Design review of the part built by this model. Coordinates are the model's own, in mm. A direction names the side the tool comes from. Coordinates: 2 decimals unless noted, no trailing zeros. Write each loop counter-clockwise with the first axis right and the second up, starting at its lowest first coordinate (ties: lowest second). Pieces come first, ordered by that corner, then holes. Notation, with made-up numbers: M 88.5,15 L 139.5,15 A20 cw 139.5,27 Z; hole C 13.25,52.5 d6. An arc over 180 degrees is marked long. Write item = value, one per line.
```python
from build123d import *

# Parameters (mm, degrees)
SKETCH001_R   = 8
PAD_DEPTH     = 4.05
SKETCH002_R   = 9.892347
SKETCH002_R_2 = 8.778396
PAD001_DEPTH  = 4.825


with BuildPart() as part:
    # Sketch001 → Pad (new body, symmetric)
    with BuildSketch(Plane.XY):
        with BuildLine():
            ThreePointArc((-12.471576, -8.239007), (5.253972, -13.993471), (14.812215, 2.004932))
            ThreePointArc((14.049591, 4.890442), (13.918155, 3.312171), (14.812215, 2.004932))
            ThreePointArc((14.049591, 4.890442), (6.504678, 10.917918), (-3.152003, 10.849328))
            ThreePointArc((-10.894672, 13.052776), (-7.942462, 8.721353), (-3.152003, 10.849328))
            Line((-10.894672, 13.052776), (-12.022041, 13.052776))
            Line((-12.022041, 13.052776), (-17.151012, 7.540552))
            Line((-17.151012, 7.540552), (-57.172882, 8.741419))
            Line((-83.948982, -1.605249), (-57.172882, 8.741419))
            Line((-82.650063, -5.462648), (-83.948982, -1.605249))
            Line((-57.419521, 2.370234), (-82.650063, -5.462648))
            Line((-20.377901, -5.481424), (-57.419521, 2.370234))
            Line((-18.078703, -9.566922), (-20.377901, -5.481424))
            Line((-12.471576, -8.239007), (-18.078703, -9.566922))
        make_face()
        Circle(SKETCH001_R, mode=Mode.SUBTRACT)
    extrude(amount=PAD_DEPTH, both=True)

    # Sketch002 → Pad001 (join, symmetric)
    with BuildSketch(Plane.XY):
        Circle(SKETCH002_R)
        Circle(SKETCH002_R_2, mode=Mode.SUBTRACT)
    extrude(amount=PAD001_DEPTH, both=True)


solid = part.part
```
Q1. For P1, Ø3, axis at y = -5, z = -1, coming from the +X side; P2, Ø5.5, axis at x = 2, y = -3.5, coming from the +Z side; P3, Ø5, axis at x = -5.5, z = 4, coming from the -Y side; P4, Ø2, axis at x = -57.5, z = 3.5, coming from the -Y side, all flat-tipped, find the tip position at first contact; note any pin that passes through.
Check result:
P1 = 14.53
P2 = through
P3 = -14.64
P4 = 2.03
Q2. Consider section D-D, the plane x = 0. State the section outline as (y, z) points (3 decimals), and give its area (3 significant figures).
Check result:
outline = M -14.947,-4.05 L -9.892,-4.05 L -9.892,-4.825 L -8.778,-4.825 L -8.778,-4.05 L -8,-4.05 L -8,4.05 L -8.778,4.05 L -8.778,4.825 L -9.892,4.825 L -9.892,4.05 L -14.947,4.05 Z; M 8,-4.05 L 8.778,-4.05 L 8.778,-4.825 L 9.892,-4.825 L 9.892,-4.05 L 11.605,-4.05 L 11.605,4.05 L 9.892,4.05 L 9.892,4.825 L 8.778,4.825 L 8.778,4.05 L 8,4.05 Z
area = 88.9 mm²
Q3. Consider section B-B, the plane y = 0. State the section outline as (x, z) points (3 decimals).
Check result:
outline = M -79.795,-4.05 L -65.054,-4.05 L -65.054,4.05 L -79.795,4.05 Z; M -46.238,-4.05 L -9.892,-4.05 L -9.892,-4.825 L -8.778,-4.825 L -8.778,-4.05 L -8,-4.05 L -8,4.05 L -8.778,4.05 L -8.778,4.825 L -9.892,4.825 L -9.892,4.05 L -46.238,4.05 Z; M 8,-4.05 L 8.778,-4.05 L 8.778,-4.825 L 9.892,-4.825 L 9.892,-4.05 L 14.947,-4.05 L 14.947,4.05 L 9.892,4.05 L 9.892,4.825 L 8.778,4.825 L 8.778,4.05 L 8,4.05 Z
Q4. Consider section C-C, the plane z = -2.25. State the section outline as (x, y) points (3 decimals).
Check result:
outline = M -83.949,-1.605 L -82.65,-5.463 L -57.42,2.37 L -20.378,-5.481 L -18.079,-9.567 L -12.472,-8.239 A14.947 ccw 14.812,2.005 A2.365 cw 14.05,4.89 A14.455 ccw -3.152,10.849 A4.091 cw -10.895,13.053 L -12.022,13.053 L -17.151,7.541 L -57.173,8.741 Z; hole C 0,0 d16
Q5. Wall thickness on line 1 (Y direction, x = 0, z = -4.4); line 2 (Z direction, x = -58.5, y = 7.75); line 3 (Y direction, x = 0, z = -2.5): over which ranges is each line inside the solid? List them lowest first.
Check result:
line_1 = -9.89 to -8.78, 8.78 to 9.89
line_2 = -4.05 to 4.05
line_3 = -14.95 to -8, 8 to 11.61
Q6. Consider section A-A, the plane y = 4. State the section outline as (x, z) points (3 decimals).
Check result:
outline = M -69.443,-4.05 L -9.048,-4.05 L -9.048,-4.825 L -7.814,-4.825 L -7.814,-4.05 L -6.928,-4.05 L -6.928,4.05 L -7.814,4.05 L -7.814,4.825 L -9.048,4.825 L -9.048,4.05 L -69.443,4.05 Z; M 6.928,-4.05 L 7.814,-4.05 L 7.814,-4.825 L 9.048,-4.825 L 9.048,-4.05 L 13.841,-4.05 L 13.841,4.05 L 9.048,4.05 L 9.048,4.825 L 7.814,4.825 L 7.814,4.05 L 6.928,4.05 Z
Q7. Machinability: for faces 1 (the flat face through (-2, -8, -4.05)), 2 (the flat face through (-2, -8, 4.05)), 3 (the cylindrical face through (13.912, 3.334, 0.057)), 4 (the cylindrical face through (6.635, 10.872, 0.057)), 5 (the flat face through (-38.64, -1.61, 0.06)), which of the approach directions +Z, -Z, +X, -X, +Y, -Y give a long, thin tool a straight path to every point of the face, cutting with its end or side? Answer none if there is none.
Check result:
face_1 = -Z
face_2 = +Z
face_3 = +Z, -Z, +X
face_4 = +Z, -Z, +Y
face_5 = +Z, -Z, -Y
Q8. The part is to be moulded in two halves that separate along Y. For faces 6 (the flat face through (-14.551, 10.335, 0.057)), 7 (the cylindrical face through (-7.85, -6.02, 4.44)), 8 (the cylindrical face through (-1.9, -8.57, -4.44)), say which applies: +Y half, -Y half, draft (parallel to the pull), parting line (faces both ways), or undercut.
Check result:
face_6 = +Y half
face_7 = parting line
face_8 = undercut
